from build123d import *

# Parameters (mm, degrees)
SKETCH2_R           = 0.75
BOSS_EXTRUDE1_DEPTH = 5
SKETCH3_W           = 0.99
SKETCH3_H           = 0.65
SKETCH4_R           = 1.17
CUT_EXTRUDE1_DEPTH  = 7.5
SKETCH5_W           = 1.13
SKETCH5_H           = 0.9


with BuildPart() as part:
    # Sketch1 → Revolve2 (revolve)
    with BuildSketch(Plane.XY):
        Polygon((0, 0), (-4.25, 0), (-4.25, 5.5), (-8.5, 5.5), (-8.5, 7), (-7.5, 7), (-7.5, 39.5), (0, 39.5), align=None)
    revolve(axis=Axis((0, 0, 0), (0, 1, 0)))

    # Sketch2 → Boss-Extrude1 (add)
    with BuildSketch(Plane(origin=(0, 39.5, 0), x_dir=(1, 0, 0), z_dir=(0, 1, 0))):
        with Locations((1.5, 4.5)):
            Circle(SKETCH2_R)
        with Locations((-1.5, 4.5)):
            Circle(SKETCH2_R)
    extrude(amount=BOSS_EXTRUDE1_DEPTH)

    # Sketch3 → Cut-Revolve1 (revolve, cut)
    with BuildSketch(Plane(origin=(0, 0, 0), x_dir=(0, 0, -1), z_dir=(1, 0, 0))):
        with Locations((3.755, 0.325)):
            Rectangle(SKETCH3_W, SKETCH3_H)
    revolve(axis=Axis((0, 0, 0), (0, 1, 0)), mode=Mode.SUBTRACT)

    # Sketch4 → Cut-Extrude1 (cut)
    with BuildSketch(Plane.XZ):
        Circle(SKETCH4_R)
    extrude(amount=-CUT_EXTRUDE1_DEPTH, mode=Mode.SUBTRACT)

    # Sketch5 → Cut-Revolve2 (revolve, cut)
    with BuildSketch(Plane(origin=(0, 0, 0), x_dir=(0, 0, -1), z_dir=(1, 0, 0))):
        with Locations((7.065, 5.95)):
            Rectangle(SKETCH5_W, SKETCH5_H)
    revolve(axis=Axis((0, 0, 0), (0, 1, 0)), mode=Mode.SUBTRACT)


solid = part.part
Build history of the part. All positions in model axes, mm. A direction names the side the tool comes from. Round coordinates to 2 decimals unless told otherwise and drop trailing zeros. Write each loop counter-clockwise with the first axis right and the second up, starting at its lowest first coordinate (ties: lowest second). Pieces come first, ordered by that corner, then holes. Notation, with made-up numbers: (33.25, -16.75) -> (81.25, -16.75) arc R6 cw to (81.25, -11.75) -> close; hole circle Ø4 at (-6, 23). An arc over 180 degrees is marked (long way). Use one line per item in the form item = value.
Q1. Two-plate mould, pull along Z, no slides. Class faces 1 (the flat face through (0, 7, -8)), 2 (the flat face through (0, 7.5, 0)), 3 (the cylindrical face through (-4.054, 3.109, 1.277)): released by +Z, released by -Z, zero draft, split by the parting line, or undercut.
Conclusion:
face_1 = zero draft
face_2 = undercut
face_3 = split by the parting line
Q2. Drill centre lines: L1, parallel to Z at x = 0, y = 5.95; L2, parallel to Z at x = -0.75, y = 6; L3, parallel to Y at x = 5, z = 0.5. Where is each one in solid material? Low to high.
Conclusion:
L1 = -8.5 to -7.63, -6.5 to -1.17, 1.17 to 6.5, 7.63 to 8.5
L2 = -8.47 to -7.59, -6.46 to -0.9, 0.9 to 6.46, 7.59 to 8.47
L3 = 5.5 to 39.5
Q3. Band-saw the part on C-C, the plane y = 27.5. Write the cut outline in (x, z), then the cut area to 3 significant figures.
Conclusion:
outline = circle Ø15 at (0, 0)
area = 177 mm²
Q4. Drop flat-ended pins along their axis: P1, Ø8, axis at x = -0.5, z = 1.5, coming from the -Y side; P2, Ø1, axis at x = -1.5, y = 6, coming from the +Z side; P3, Ø8, axis at y = 16, z = 4, coming from the +X side; P4, Ø6, axis at x = -4.5, z = -0.5, coming from the +Y side. Give the stop position or say it passes through.
Conclusion:
P1 = 0
P2 = 8.44
P3 = 7.5
P4 = 39.5
Q5. Band-saw the part on B-B, the plane x = 0. Write the cut outline in (y, z).
Conclusion:
outline = (0, -3.26) -> (0.65, -3.26) -> (0.65, -4.25) -> (5.5, -4.25) -> (5.5, -6.5) -> (6.4, -6.5) -> (6.4, -7.63) -> (5.5, -7.63) -> (5.5, -8.5) -> (7, -8.5) -> (7, -7.5) -> (39.5, -7.5) -> (39.5, 7.5) -> (7, 7.5) -> (7, 8.5) -> (5.5, 8.5) -> (5.5, 7.63) -> (6.4, 7.63) -> (6.4, 6.5) -> (5.5, 6.5) -> (5.5, 4.25) -> (0.65, 4.25) -> (0.65, 3.26) -> (0, 3.26) -> (0, 1.17) -> (7.5, 1.17) -> (7.5, -1.17) -> (0, -1.17) -> close
Q6. Tool access for faces 4 (the flat face through (-1.5, 44.5, -4.5)), 5 (the cylindrical face through (1.337, 41.965, -3.768)), 6 (the flat face through (-6, 5.5, 5)): list every direction of +Z, -Z, +X, -X, +Y, -Y with a clear straight run to the whole face (end or side of a thin tool).
Conclusion:
face_4 = +Z, -Z, +X, -X, +Y
face_5 = +Y
face_6 = -Y
Q7. Band-saw the part on A-A, the plane z = 0. Write the cut outline in (x, y), then the cut area to 3 significant figures.
Conclusion:
outline = (-8.5, 5.5) -> (-7.63, 5.5) -> (-7.63, 6.4) -> (-6.5, 6.4) -> (-6.5, 5.5) -> (-4.25, 5.5) -> (-4.25, 0.65) -> (-3.26, 0.65) -> (-3.26, 0) -> (-1.17, 0) -> (-1.17, 7.5) -> (1.17, 7.5) -> (1.17, 0) -> (3.26, 0) -> (3.26, 0.65) -> (4.25, 0.65) -> (4.25, 5.5) -> (6.5, 5.5) -> (6.5, 6.4) -> (7.63, 6.4) -> (7.63, 5.5) -> (8.5, 5.5) -> (8.5, 7) -> (7.5, 7) -> (7.5, 39.5) -> (-7.5, 39.5) -> (-7.5, 7) -> (-8.5, 7) -> close
area = 539 mm²
Q8. Band-saw the part on D-D, the plane z = 2.75. Write the cut outline in (x, y).
Conclusion:
outline = (-8.04, 5.5) -> (-7.12, 5.5) -> (-7.12, 6.4) -> (-5.89, 6.4) -> (-5.89, 5.5) -> (-3.24, 5.5) -> (-3.24, 0.65) -> (-1.75, 0.65) -> (-1.75, 0) -> (1.75, 0) -> (1.75, 0.65) -> (3.24, 0.65) -> (3.24, 5.5) -> (5.89, 5.5) -> (5.89, 6.4) -> (7.12, 6.4) -> (7.12, 5.5) -> (8.04, 5.5) -> (8.04, 7) -> (6.98, 7) -> (6.98, 39.5) -> (-6.98, 39.5) -> (-6.98, 7) -> (-8.04, 7) -> close
